Input: part model. Units: mm. Frame: model coordinates. Coordinates: 2 decimals unless noted, no trailing zeros. Loops run counter-clockwise (first coordinate to the right, second up) from the corner with the lowest first, then second, coordinate; pieces in that order, holes last. Notation, with made-up numbers: (0.5, 61.25) -> (28.5, 61.25) arc R17 ccw to (28.5, 86.25) -> close; hole circle Ø9 at (19.5, -9.5). An arc over 180 degrees is marked (long way). Answer as a JSON object with one key per item and string values.
from build123d import *

# Parameters (mm, degrees)
SKETCH1_R           = 75
BOSS_EXTRUDE1_DEPTH = 100
SKETCH2_OUTSIDE_W   = 198.904
SKETCH2_OUTSIDE_H   = 198.904
SKETCH2_OUTSIDE_W_2 = 44.4
SKETCH2_OUTSIDE_H_2 = 99.351371604
CUT_EXTRUDE1_DEPTH  = 146.773797371
SKETCH3_W           = 44.4
SKETCH3_H           = 53.109155611
CUT_EXTRUDE2_DEPTH  = 143.70085858
SKETCH4_R           = 18.4
CUT_EXTRUDE3_DEPTH  = 82.472603048


with BuildPart() as part:
    # Sketch1 → Boss-Extrude1 (new body)
    with BuildSketch(Plane(origin=(0, 0, 0), x_dir=(1, 0, 0), z_dir=(0, 1, 0))):
        with Locations(Location((0, 0, 0), (0, 0, 270))):
            Circle(SKETCH1_R)
    extrude(amount=BOSS_EXTRUDE1_DEPTH)

    # Sketch2 outside → Cut-Extrude1 (cut, through all)
    with BuildSketch(Plane(origin=(0, 100, 0), x_dir=(1, 0, 0), z_dir=(0, 1, 0))):
        Rectangle(SKETCH2_OUTSIDE_W, SKETCH2_OUTSIDE_H)
        Rectangle(SKETCH2_OUTSIDE_W_2, SKETCH2_OUTSIDE_H_2, mode=Mode.SUBTRACT)
    extrude(amount=-CUT_EXTRUDE1_DEPTH, mode=Mode.SUBTRACT)

    # Sketch3 → Cut-Extrude2 (cut, through all)
    with BuildSketch(Plane.XY.offset(49.675685802)):
        with Locations((0, 73.445422194)):
            Rectangle(SKETCH3_W, SKETCH3_H)
    extrude(amount=-CUT_EXTRUDE2_DEPTH, mode=Mode.SUBTRACT)

    # Sketch4 → Cut-Extrude3 (cut, through all)
    with BuildSketch(Plane.ZY.offset(22.2)):
        with Locations((26.675685802, 21.890844389)):
            Circle(SKETCH4_R)
        with Locations((-26.675685802, 21.890844389)):
            Circle(SKETCH4_R)
    extrude(amount=-CUT_EXTRUDE3_DEPTH, mode=Mode.SUBTRACT)


solid = part.part
1. Line query: line 1 along Z through (x, y) = (0, 22); line 2 along Z through (x, y) = (17.5, 10.5); line 3 along Y through (x, z) = (-1, -14.5). Output: solid intervals per line, ascending.
Reply:
{"line 1": "z = -49.68 to -45.08, -8.28 to 8.28, 45.08 to 49.68", "line 2": "z = -49.68 to -41.13, -12.23 to 12.23, 41.13 to 49.68", "line 3": "y = 0 to 8.1, 35.69 to 46.89"}
2. Section query A-A (z = -15.5). Return loops of the section in (x, y), plus the area to 3 significant figures.
Reply:
{"outline": "(-22.2, 0) -> (22.2, 0) -> (22.2, 7.27) -> (-22.2, 7.27) -> close; (-22.2, 36.51) -> (22.2, 36.51) -> (22.2, 46.89) -> (-22.2, 46.89) -> close", "area": "784 mm2"}
3. Pin query (flat end, axial travel): P1, Ø1, axis at y = 5.5, z = -26.5, coming from the -X side. Return the tip coordinate at first contact, or that it passes through.
Reply:
{"P1": "passes through"}
4. Mould query, pull axis Y, two halves, no side actions, for faces 1 (the face through (0, 0, -1)), 2 (the face through (0, 46.891, 1)), 3 (the face through (0, 24, 49.676)), 4 (the face through (-0.311, 37.406, 36.567)). Classes: pulls with the +Y half, pulls with the -Y half, needs draft (parallel to the pull), parting line crosses it, or undercut.
Reply:
{"face 1": "pulls with the -Y half", "face 2": "pulls with the +Y half", "face 3": "needs draft", "face 4": "undercut"}
5. Section query C-C (x = -12). Return loops of the section in (y, z).
Reply:
{"outline": "(0, -49.68) -> (46.89, -49.68) -> (46.89, 49.68) -> (0, 49.68) -> close; hole circle Ø36.8 at (21.89, -26.68); hole circle Ø36.8 at (21.89, 26.68)"}
6. Section query B-B (y = 16.5). Return loops of the section in (x, z).
Reply:
{"outline": "(-22.2, -49.68) -> (22.2, -49.68) -> (22.2, -44.27) -> (-22.2, -44.27) -> close; (-22.2, -9.08) -> (22.2, -9.08) -> (22.2, 9.08) -> (-22.2, 9.08) -> close; (-22.2, 44.27) -> (22.2, 44.27) -> (22.2, 49.68) -> (-22.2, 49.68) -> close"}
7. Section query D-D (z = 27). Return loops of the section in (x, y), plus the area to 3 significant figures.
Reply:
{"outline": "(-22.2, 0) -> (22.2, 0) -> (22.2, 3.49) -> (-22.2, 3.49) -> close; (-22.2, 40.29) -> (22.2, 40.29) -> (22.2, 46.89) -> (-22.2, 46.89) -> close", "area": "448 mm2"}
